Here's how the part is built. I have some questions about the finished solid (model axes, mm). A direction names the side the tool comes from. Coordinates: 2 decimals unless noted, no trailing zeros. Order: outer loops, then holes, each group sorted by start corner. A loop starts at its lowest first (then second) coordinate and runs counter-clockwise, first axis right, second up. Notation, with made-up numbers: M 46,45 L 70,45 A26 cw 70,64 Z; hole C -8.75,5.25 d3. An arc over 180 degrees is marked long. One line per question, with ' | ' between items. Start each with the question number.
Autodesk Inventor part; units mm, degrees
ref_plane "YZ Plane" through (0, 0, 0) normal (1, 0, 0) x (0, 1, 0)
ref_plane "XZ Plane" through (0, 0, 0) normal (0, 1, 0) x (-1, 0, 0)
ref_plane "XY Plane" through (0, 0, 0) normal (0, 0, 1) x (1, 0, 0)
sketch "スケッチ1" plane through (0, 0, 0) normal (1, 0, 0) x (0, 1, 0)
  line L0 (-12.5, 0) -> (12.5, 0)
  line L1 (0, 0) -> (0, 3.1754) construction
  line L2 (-12.2544, 3.1754) -> (-12.5, 2.75)
  line L3 (-12.5, 2.75) -> (-12.5, 0)
  line L4 (-12.2544, 3.1754) -> (12.2544, 3.1754)
  line L5 (12.2544, 3.1754) -> (12.5, 2.75)
  line L6 (12.5, 2.75) -> (12.5, 0)
  dimension "d1" = 2.75
  dimension "d2" = 3.1754
  dimension "d3" = 30
  dimension "d4" = 25
revolve "回転1" add sketch "スケッチ1" angle 360 about axis through (0, -12.5, 0) along (0, 1, 0)
sketch "スケッチ2" plane through (0, 12.5, 0) normal (0, 1, 0) x (1, 0, 0)
  line L0 (0, -3.1754) -> (-2.75, -1.5877)
  line L1 (-2.75, -1.5877) -> (-2.75, 1.5877)
  line L2 (-2.75, 1.5877) -> (0, 3.1754)
  line L3 (0, 3.1754) -> (2.75, 1.5877)
  line L4 (2.75, 1.5877) -> (2.75, -1.5877)
  line L5 (2.75, -1.5877) -> (0, -3.1754)
  circle A0 centre (0, 0) radius 3.1754
  point P0 (0, 0)
  point P1 (0, 0)
  point P2 (0, 0)
  point P3 (0, 0)
  point P4 (0, 3.1754)
  point P5 (0, 3.1754)
  point P6 (2.75, -1.5877)
  point P7 (2.75, -1.5877)
extrude "押し出し1" cut sketch "スケッチ2" against normal through all contours A0 L0 | L5 A0 | A0 L1 | L4 A0 | A0 L2 | L3 A0
hole "穴1" at (0, 12.5, 0) direction (0, -1, 0) diameter 2.459 depth 3.3 tip angle 118 countersink diameter 3 countersink angle 90
mirror "Mirror1" about plane through (0, 0, 0) normal (0, 1, 0) of "穴1"
equation "\"d2\" = 1.1547 * d1"
properties part number "BSL-325BE" material "Aluminum 2014-T4"
1. We'd pull the mould along Z, two halves only. Please class faces 1 (the face through (-2.525, 12.404, 1.46)), 2 (the face through (-0.064, -8.59, 0.204)), 3 (the face through (-1.2, -12.5, 1.2)): released by +Z, released by -Z, zero draft, split by the parting line, or undercut.
2. Imagine slicing it at A-A (y = 10). List the corners of the cut face in (x, z) for me, then the cut area to 3 significant figures.
3. Which directions (+Z, -Z, +X, -X, +Y, -Y) give clear straight access to the entire face, cutting with the end or side of a thin tool? Please do faces 4 (the face through (-2.52, 12.41, -1.44)), 5 (the face through (0.748, 10.694, -0.976)), 6 (the face through (-0.748, -10.694, -0.976)).
4. I need wall thicknesses on line 1 (X direction, y = 10.6, z = 0); line 2 (Z direction, x = -0.45, y = -10.25); line 3 (Z direction, x = -0.1, y = -7.25). Which ranges of each line are inside material? Lowest first, please.
5. Imagine slicing it at B-B (y = -2.25). List the corners of the cut face in (x, z) for me, then the cut area to 3 significant figures.
6. Will these pins go through, and if not, where does the flat tip stop? pin 1 (1.5 mm diameter, centred on x = 2, z = 2, fed in from -Y); pin 2 (1.5 mm diameter, centred on x = 0, z = 0, fed in from -Y); pin 3 (2 mm diameter, centred on x = 0, z = 0, fed in from -Y); pin 4 (1.5 mm diameter, centred on x = 1.5, y = -2, fed in from -Z).
Entries:
1) face 1: released by +Z | face 2: undercut | face 3: zero draft
2) outline: M -2.75,-1.59 L 0,-3.18 L 2.75,-1.59 L 2.75,1.59 L 0,3.18 L -2.75,1.59 Z; hole C 0,0 d2.46 | area: 21.4 mm²
3) face 4: -Z, -X, +Y | face 5: +Y | face 6: -Y
4) line 1: -2.75 to -1.23, 1.23 to 2.75 | line 2: -2.92 to -1.14, 1.14 to 2.92 | line 3: -3.12 to 3.12
5) outline: M -2.75,-1.59 L 0,-3.18 L 2.75,-1.59 L 2.75,1.59 L 0,3.18 L -2.75,1.59 Z | area: 26.2 mm²
6) pin 1: y = -12.5 | pin 2: y = -8.91 | pin 3: y = -9.06 | pin 4: z = -2.74
